Print and shaded views of the part. All mm, measured from the part's lowest x, y and z. Round coordinates to 2 decimals unless told otherwise and drop trailing zeros. Write each loop counter-clockwise with the first axis right and the second up, starting at its lowest first coordinate (ties: lowest second). Pieces come first, ordered by that corner, then holes.
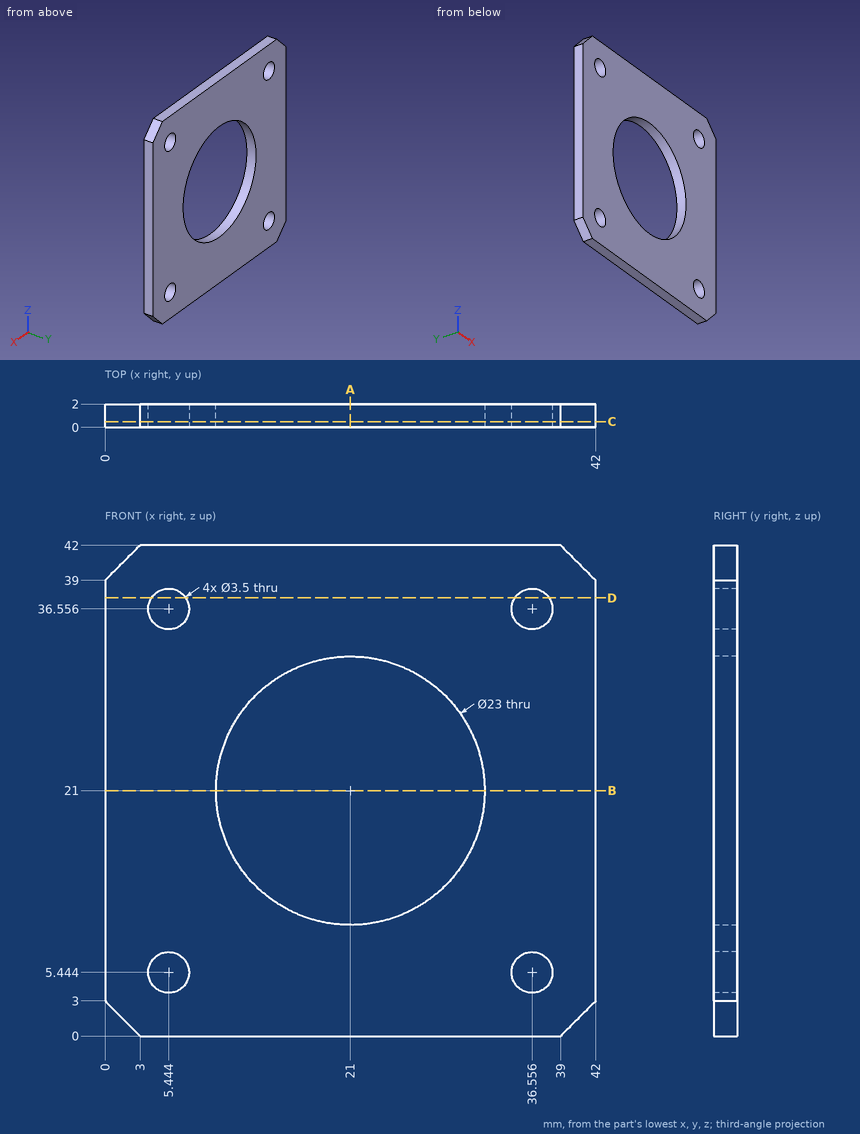
1) Slice it at D-D (z = 37.5). Write the cut outline in (x, y).
Results:
outline: (0, 0) - (3.97, 0) - (3.97, 2) - (0, 2) - close; (6.92, 0) - (35.08, 0) - (35.08, 2) - (6.92, 2) - close; (38.03, 0) - (42, 0) - (42, 2) - (38.03, 2) - close
2) Slice it at B-B (z = 21). Write the cut outline in (x, y), plus the area to 3 significant figures.
Results:
outline: (0, 0) - (9.5, 0) - (9.5, 2) - (0, 2) - close; (32.5, 0) - (42, 0) - (42, 2) - (32.5, 2) - close
area: 38.0 mm2
3) Slice it at A-A (x = 21). Write the cut outline in (y, z), plus the area to 3 significant figures.
Results:
outline: (0, 0) - (2, 0) - (2, 9.5) - (0, 9.5) - close; (0, 32.5) - (2, 32.5) - (2, 42) - (0, 42) - close
area: 38.0 mm2
4) Wall check: L1, parallel to X at y = 0.6, z = 37; L2, parallel to X at y = 0.8, z = 21.5; L3, parallel to Z at x = 4, y = 1.2 (1 decimal). Give the ranges that are in metal, low to high.
Results:
L1: x = 0 to 3.75, 7.14 to 34.86, 38.25 to 42
L2: x = 0 to 9.51, 32.49 to 42
L3: z = 0 to 4.5, 6.4 to 35.6, 37.5 to 42
5) Slice it at C-C (y = 0.5). Write the cut outline in (x, z).
Results:
outline: (0, 3) - (3, 0) - (39, 0) - (42, 3) - (42, 39) - (39, 42) - (3, 42) - (0, 39) - close; hole circle Ø3.5 at (5.44, 5.44); hole circle Ø3.5 at (5.44, 36.56); hole circle Ø23 at (21, 21); hole circle Ø3.5 at (36.56, 5.44); hole circle Ø3.5 at (36.56, 36.56)
